```python
from build123d import *

# Parameters (mm, degrees)
SKETCH1_R           = 30
SKETCH1_R_2         = 10
SKETCH1_R_3         = 1.45
BOSS_EXTRUDE1_DEPTH = 5
SKETCH2_W           = 20
SKETCH2_H           = 14.5
BOSS_EXTRUDE2_DEPTH = 5
SKETCH3_W           = 20
SKETCH3_H           = 113.5
BOSS_EXTRUDE3_DEPTH = 6
SKETCH4_W           = 20
SKETCH4_H           = 14.5
SKETCH4_R           = 1.7
BOSS_EXTRUDE4_DEPTH = 4


with BuildPart() as part:
    # Sketch1 → Boss-Extrude1 (new body)
    with BuildSketch(Plane.XY.offset(384.5)):
        with Locations((300, 300)):
            Circle(SKETCH1_R)
        with Locations((300, 300)):
            Circle(SKETCH1_R_2, mode=Mode.SUBTRACT)
        with Locations((286.774831823, 318.202882373)):
            Circle(SKETCH1_R_3, mode=Mode.SUBTRACT)
        with Locations((278.601228383, 293.047117627)):
            Circle(SKETCH1_R_3, mode=Mode.SUBTRACT)
        with Locations((300, 277.5)):
            Circle(SKETCH1_R_3, mode=Mode.SUBTRACT)
        with Locations((321.398771617, 293.047117627)):
            Circle(SKETCH1_R_3, mode=Mode.SUBTRACT)
        with Locations((313.225168177, 318.202882373)):
            Circle(SKETCH1_R_3, mode=Mode.SUBTRACT)
    extrude(amount=BOSS_EXTRUDE1_DEPTH)

    # Sketch2 → Boss-Extrude2 (add)
    with BuildSketch(Plane.XY.offset(384.5)):
        with Locations((300, 327.25)):
            Rectangle(SKETCH2_W, SKETCH2_H)
    extrude(amount=BOSS_EXTRUDE2_DEPTH)

    # Sketch3 → Boss-Extrude3 (add)
    with BuildSketch(Plane(origin=(0, 328.5, 0), x_dir=(1, 0, 0), z_dir=(0, 1, 0))):
        with Locations((300, -332.75)):
            Rectangle(SKETCH3_W, SKETCH3_H)
    extrude(amount=BOSS_EXTRUDE3_DEPTH)

    # Sketch4 → Boss-Extrude4 (add)
    with BuildSketch(Plane.XY.offset(276)):
        with Locations((300, 327.25)):
            Rectangle(SKETCH4_W, SKETCH4_H)
        with Locations((295, 324)):
            Circle(SKETCH4_R, mode=Mode.SUBTRACT)
        with Locations((305, 324)):
            Circle(SKETCH4_R, mode=Mode.SUBTRACT)
    extrude(amount=BOSS_EXTRUDE4_DEPTH)


solid = part.part
```
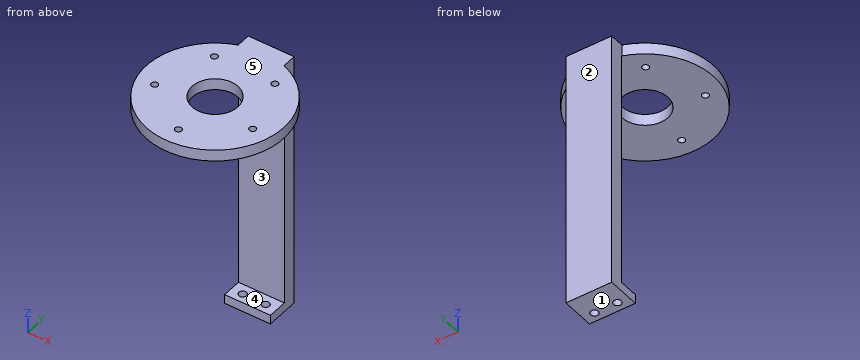
Can you work these out from the model? Positions are in its coordinate system, mm. Face numbers are marked on the shaded views. A direction names the side the tool comes from. Coordinates: 2 decimals unless noted, no trailing zeros. Order: outer loops, then holes, each group sorted by start corner. A loop starts at its lowest first (then second) coordinate and runs counter-clockwise, first axis right, second up.
1. I'm going to push flat-ended pins straight in: pin 1 (10 mm diameter, centred on x = 301.5, z = 345, fed in from -Y); pin 2 (1.7 mm diameter, centred on x = 313.23, y = 318.2, fed in from +Z); pin 3 (11.5 mm diameter, centred on y = 326, z = 348.5, fed in from -X); pin 4 (4.5 mm diameter, centred on y = 331, z = 341.5, fed in from +X). Where does each tip first touch, or does it pass through?
2. Thinking about a two-plate mould opening in Z: for the marked faces 1, 2 and 3, which applies, +Z half, -Z half, draft (parallel to the pull), parting line (faces both ways), or undercut?
3. If we section it at B-B (y = 324): Please give me the cut outline in (x, z), then the cut area to 3 significant figures.
4. If we section it at D-D (z = 319): Please give me the cut outline in (x, y), then the cut area to 3 significant figures.
5. For the marked faces 4 and 5, which set-ups out of +Z, -Z, +X, -X, +Y, -Y let a thin tool reach every point of the face, with its end or its side?
6. If we section it at A-A (y = 300): Please give me the cut outline in (x, z), then the cut area to 3 significant figures.
7. If we section it at C-C (x = 295): Please give me the cut outline in (y, z), then the cut area to 3 significant figures.
8. I need wall thicknesses on line 1 (Y direction, x = 300, z = 386.95); line 2 (Y direction, x = 305, z = 277.4); line 3 (Z direction, x = 299, y = 324). Which ranges of each line are inside material? Lowest first, please.
Entries:
1. pin 1: stops at y = 328.5
1. pin 2: passes through
1. pin 3: stops at x = 290
1. pin 4: stops at x = 310
2. face 1: -Z half
2. face 2: draft
2. face 3: undercut
3. outline: (282, 384.5) - (318, 384.5) - (318, 389.5) - (282, 389.5) - close; (290, 276) - (293.3, 276) - (293.3, 280) - (290, 280) - close; (296.7, 276) - (303.3, 276) - (303.3, 280) - (296.7, 280) - close; (306.7, 276) - (310, 276) - (310, 280) - (306.7, 280) - close
3. area: 233 mm2
4. outline: (290, 328.5) - (310, 328.5) - (310, 334.5) - (290, 334.5) - close
4. area: 120 mm2
5. face 4: +X, -X, -Y
5. face 5: +Z, +X, -X, +Y, -Y
6. outline: (270, 384.5) - (290, 384.5) - (290, 389.5) - (270, 389.5) - close; (310, 384.5) - (330, 384.5) - (330, 389.5) - (310, 389.5) - close
6. area: 200 mm2
7. outline: (270.42, 384.5) - (291.34, 384.5) - (291.34, 389.5) - (270.42, 389.5) - close; (308.66, 384.5) - (328.5, 384.5) - (328.5, 280) - (325.7, 280) - (325.7, 276) - (334.5, 276) - (334.5, 389.5) - (308.66, 389.5) - close; (320, 276) - (322.3, 276) - (322.3, 280) - (320, 280) - close
7. area: 905 mm2
8. line 1: y = 270 to 276.05, 278.95 to 290, 310 to 334.5
8. line 2: y = 320 to 322.3, 325.7 to 334.5
8. line 3: z = 276 to 280, 384.5 to 389.5
